Source: CAD feature listing. Evaluate the final solid. Frame: model axes, mm. Face numbers are marked on the shaded views. Coordinates: 2 decimals unless noted, no trailing zeros. Loops run counter-clockwise (first coordinate to the right, second up) from the corner with the lowest first, then second, coordinate; pieces in that order, holes last.
Item 1: Pull-direction query (Y, two-part tool) for the marked faces 1 and 2; classes: +Y half, -Y half, draft (parallel to the pull), parting line (faces both ways), or undercut.
Item 2: Line query: probe 1 along X at (y, z) = (-1849, 8); probe 2 along Y at (x, z) = (1797, 7.5); probe 3 along Y at (x, z) = (1770, 1). Output: solid intervals per line, ascending.
Item 3: Section query B-B, the plane z = 3.5. State how many separate pieces and enclosed holes the cut face has, then the cut area to 3 significant figures.
Item 4: Section query A-A, the plane x = 1814. Return the cut outline in (y, z).
Item 5: Pin query (flat end, axial travel): pin 1 Ø3 at (x, y) = (1780.42, -1800.75) entering from -Z; pin 2 Ø8 at (x, y) = (1801.5, -1752) entering from +Z; pin 3 Ø1 at (x, z) = (1791.5, 8.5) entering from +Y; pin 4 Ø7.5 at (x, y) = (1760.42, -1886.07) entering from +Z. Return the tip coordinate at first contact, or that it passes through.
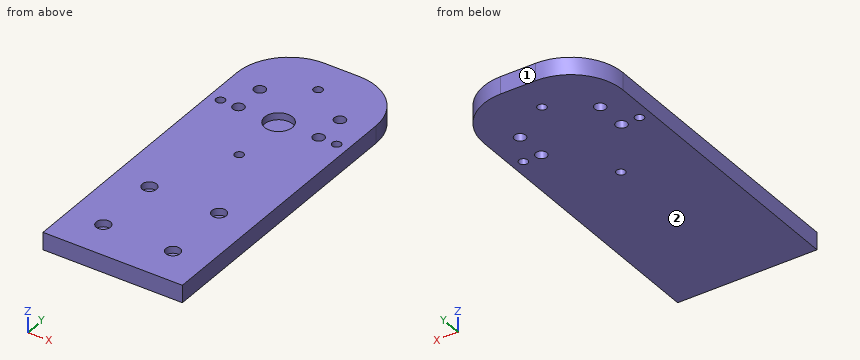
```python
from build123d import *

# Parameters (mm, degrees)
SKETCH1_W                = 80
SKETCH1_H                = 193.756044748
BOSS_EXTRUDE1_DEPTH      = 10
SCHIZZO2_R               = 2.549999997
SCHIZZO2_R_2             = 2.55
TAGLIO_ESTRUSIONE4_DEPTH = 2637.837278588
SCHIZZO3_R               = 3.25
TAGLIO_ESTRUSIONE5_DEPTH = 2637.837278588
SCHIZZO6_R               = 4.1
TAGLIO_ESTRUSIONE6_DEPTH = 4
RACCORDO1_R              = 30
SCHIZZO7_R               = 8
TAGLIO_ESTRUSIONE7_DEPTH = 4


with BuildPart() as part:
    # Sketch1 → Boss-Extrude1 (new body)
    with BuildSketch(Plane.XY):
        with Locations((1780.42117355, -1810.70620503)):
            Rectangle(SKETCH1_W, SKETCH1_H)
    extrude(amount=BOSS_EXTRUDE1_DEPTH)

    # Schizzo2 → Taglio-Estrusione4 (cut, through all)
    with BuildSketch(Plane.XY.offset(10)):
        with Locations((1747.088159885, -1767.419409113)):
            Circle(SCHIZZO2_R)
        with Locations((1780.42117355, -1734.086395448)):
            Circle(SCHIZZO2_R_2)
        with Locations((1813.754187215, -1767.419409113)):
            Circle(SCHIZZO2_R_2)
        with Locations((1780.42117355, -1800.752422779)):
            Circle(SCHIZZO2_R_2)
    extrude(amount=-TAGLIO_ESTRUSIONE4_DEPTH, mode=Mode.SUBTRACT)

    # Schizzo3 → Taglio-Estrusione5 (cut, through all)
    with BuildSketch(Plane.XY.offset(10)):
        with Locations((1803.421173548, -1749.419409113)):
            Circle(SCHIZZO3_R)
        with Locations((1803.421173548, -1767.419409113)):
            Circle(SCHIZZO3_R)
        with Locations((1757.421173548, -1749.419409113)):
            Circle(SCHIZZO3_R)
        with Locations((1757.421173548, -1767.419409113)):
            Circle(SCHIZZO3_R)
    extrude(amount=-TAGLIO_ESTRUSIONE5_DEPTH, mode=Mode.SUBTRACT)

    # Schizzo6 → Taglio-Estrusione6 (cut)
    with BuildSketch(Plane.XY.offset(10)):
        with Locations((1760.42117355, -1847.116784923)):
            Circle(SCHIZZO6_R)
        with Locations((1800.42117355, -1847.116784923)):
            Circle(SCHIZZO6_R)
        with Locations(Location((1800.42117355, -1886.070299533, 0), (0, 0, 180))):
            Circle(SCHIZZO6_R)
        with Locations(Location((1760.42117355, -1886.070299533, 0), (0, 0, 180))):
            Circle(SCHIZZO6_R)
    extrude(amount=-TAGLIO_ESTRUSIONE6_DEPTH, mode=Mode.SUBTRACT)

    # Raccordo1
    raccordo1_edges = [part.edges().sort_by_distance(p)[0] for p in [
        (1740.42117355, -1713.828182656, 5),
        (1820.42117355, -1713.828182656, 5),
    ]]
    fillet(raccordo1_edges, radius=RACCORDO1_R)

    # Schizzo7 → Taglio-Estrusione7 (cut)
    with BuildSketch(Plane.XY.offset(10)):
        with Locations((1780.42117355, -1767.419409113)):
            Circle(SCHIZZO7_R)
    extrude(amount=-TAGLIO_ESTRUSIONE7_DEPTH, mode=Mode.SUBTRACT)


solid = part.part
```
Verdict:
1. face 1: +Y half
1. face 2: draft
2. probe 1: x = 1740.42 to 1756.78, 1764.06 to 1796.78, 1804.06 to 1820.42
2. probe 2: y = -1907.58 to -1888.33, -1883.81 to -1849.38, -1844.86 to -1714.56
2. probe 3: y = -1907.58 to -1713.83
3. separate pieces: 1
3. enclosed holes: 8
3. area: 14,900 mm2
4. outline: (-1907.58, 0) - (-1769.96, 0) - (-1769.96, 10) - (-1907.58, 10) - close; (-1764.88, 0) - (-1725.28, 0) - (-1725.28, 10) - (-1764.88, 10) - close
5. pin 1: passes through
5. pin 2: stops at z = 10
5. pin 3: stops at y = -1713.83
5. pin 4: stops at z = 6
